Geometry check sheet. Reference: the model listing, model coordinates, mm. A direction names the side the tool comes from. Coordinates: 2 decimals unless noted, no trailing zeros. Write each loop counter-clockwise with the first axis right and the second up, starting at its lowest first coordinate (ties: lowest second). Pieces come first, ordered by that corner, then holes. Notation, with made-up numbers: (30.25, 39) -> (57.25, 39) arc R22 ccw to (57.25, 56) -> close; hole circle Ø11 at (64.5, 68.5). An arc over 180 degrees is marked (long way). Put each result on its own line as item: value. Start each with the question number.
from build123d import *

# Parameters (mm, degrees)
SKETCH3_R          = 1.7
CUT_EXTRUDE1_DEPTH = 68.372101051
CIRPATTERN1_COUNT  = 4
SKETCH4_R          = 2.95
CUT_EXTRUDE2_DEPTH = 3
CIRPATTERN2_COUNT  = 4


with BuildPart() as part:
    # Sketch1 → Revolve1 (revolve)
    with BuildSketch(Plane.XY):
        Polygon((25, 0), (47, 0), (47, -5), (35, -5), (35, -11), (25, -11), align=None)
    revolve(axis=Axis((0, -62.255842479, 0), (0, 1, 0)))

    # Sketch3 → Cut-Extrude1 (cut, symmetric)
    with BuildSketch(Plane(origin=(0, 0, 0), x_dir=(1, 0, 0), z_dir=(0, 1, 0))):
        with Locations(Location((0, 30, 0), (0, 0, 180))):
            Circle(SKETCH3_R)
    cut_extrude1 = extrude(amount=CUT_EXTRUDE1_DEPTH, both=True, mode=Mode.SUBTRACT)

    # CirPattern1: Cut-Extrude1 ×4 about axis
    cirpattern1_axis = Axis((0, 0, 0), (0, 1, 0))
    for i in range(1, CIRPATTERN1_COUNT):
        add(cut_extrude1.rotate(cirpattern1_axis, i * 360 / CIRPATTERN1_COUNT), mode=Mode.SUBTRACT)

    # Sketch4 → Cut-Extrude2 (cut)
    with BuildSketch(Plane(origin=(0, 0, 0), x_dir=(1, 0, 0), z_dir=(0, 1, 0))):
        with Locations(Location((0, 30, 0), (0, 0, 180))):
            Circle(SKETCH4_R)
    cut_extrude2 = extrude(amount=-CUT_EXTRUDE2_DEPTH, mode=Mode.SUBTRACT)

    # CirPattern2: Cut-Extrude2 ×4 about axis
    cirpattern2_axis = Axis((0, 0, 0), (0, 1, 0))
    for i in range(1, CIRPATTERN2_COUNT):
        add(cut_extrude2.rotate(cirpattern2_axis, i * 360 / CIRPATTERN2_COUNT), mode=Mode.SUBTRACT)


solid = part.part
Item 1: Section check B-B, the plane z = 0. Enter the section's corners in (x, y), and give its area (3 significant figures).
Item 2: Section check A-A, the plane x = 0. Enter the section's corners in (y, z), and give its area (3 significant figures).
Item 3: Go/stop test with flat-tipped pins: P1, Ø1, axis at y = -6, z = 26.5, coming from the -X side; P2, Ø4, axis at y = -6, z = 29, coming from the -X side; P3, Ø1.5, axis at x = -24, y = -7.5, coming from the -Z side; P4, Ø2.5, axis at x = 30, z = 0, coming from the +Y side. Record where each tip stops, or that it passes through.
Item 4: Section check C-C, the plane y = -1.5. Enter the section's corners in (x, z), and give its area (3 significant figures).
Item 5: Mould release check, pull along X, two halves, no side actions. Record for faces 1 (the flat face through (30, -3, -2)), 2 (the flat face through (23, -11, -11)), 3 (the cylindrical face through (-28, -8, 21)), 4 (the cylindrical face through (-27.513, -1.479, 1.586)): released by +X, released by -X, zero draft, split by the parting line, or undercut.
Item 6: Access from +Z, -Z, +X, -X, +Y, -Y to the whole of each face (thin tool, end or side, straight path). Record for faces 5 (the flat face through (-35, -5, 3.3)), 6 (the cylindrical face through (27.513, -1.479, -1.586)), 7 (the cylindrical face through (44.83, -2.54, -14.12)).
Item 7: Scan lines: line 1 along Z through (x, y) = (0, -1.3); line 2 along Z through (x, y) = (0, -8). Record each from-to range of solid material in increasing order. Write a range as [from, to].
Item 8: Section check D-D, the plane x = -14. Enter the section's corners in (y, z).
From the geometry:
1. outline: (-47, -5) -> (-35, -5) -> (-35, -11) -> (-31.7, -11) -> (-31.7, -3) -> (-32.95, -3) -> (-32.95, 0) -> (-47, 0) -> close; (-28.3, -11) -> (-25, -11) -> (-25, 0) -> (-27.05, 0) -> (-27.05, -3) -> (-28.3, -3) -> close; (25, -11) -> (28.3, -11) -> (28.3, -3) -> (27.05, -3) -> (27.05, 0) -> (25, 0) -> close; (31.7, -11) -> (35, -11) -> (35, -5) -> (47, -5) -> (47, 0) -> (32.95, 0) -> (32.95, -3) -> (31.7, -3) -> close
1. area: 250 mm²
2. outline: (-11, -35) -> (-5, -35) -> (-5, -47) -> (0, -47) -> (0, -32.95) -> (-3, -32.95) -> (-3, -31.7) -> (-11, -31.7) -> close; (-11, -28.3) -> (-3, -28.3) -> (-3, -27.05) -> (0, -27.05) -> (0, -25) -> (-11, -25) -> close; (-11, 25) -> (0, 25) -> (0, 27.05) -> (-3, 27.05) -> (-3, 28.3) -> (-11, 28.3) -> close; (-11, 31.7) -> (-3, 31.7) -> (-3, 32.95) -> (0, 32.95) -> (0, 47) -> (-5, 47) -> (-5, 35) -> (-11, 35) -> close
2. area: 250 mm²
3. P1: x = -23.43
3. P2: x = -38.28
3. P3: z = -26.16
3. P4: through
4. outline: circle Ø94 at (0, 0); hole circle Ø5.9 at (-30, 0); hole circle Ø50 at (0, 0); hole circle Ø5.9 at (0, -30); hole circle Ø5.9 at (0, 30); hole circle Ø5.9 at (30, 0)
4. area: 4,870 mm²
5. face 1: undercut
5. face 2: zero draft
5. face 3: split by the parting line
5. face 4: undercut
6. face 5: -Y
6. face 6: +Y
6. face 7: +Y, -Y
7. line 1: [-47, -32.95], [-27.05, -25], [25, 27.05], [32.95, 47]
7. line 2: [-35, -31.7], [-28.3, -25], [25, 28.3], [31.7, 35]
8. outline: (-11, -32.08) -> (-5, -32.08) -> (-5, -44.87) -> (0, -44.87) -> (0, -20.71) -> (-11, -20.71) -> close; (-11, 20.71) -> (0, 20.71) -> (0, 44.87) -> (-5, 44.87) -> (-5, 32.08) -> (-11, 32.08) -> close
